from build123d import *

# Parameters (mm, degrees)
SKETCH5_W            = 10
SKETCH5_H            = 100
BOSS_EXTRUDE5_DEPTH  = 3
M3_CLEARANCE_HOLE1_D = 3.6
SKETCH8_R            = 1.75
CUT_EXTRUDE1_DEPTH   = 249.962542564
SKETCH10_W           = 10
SKETCH10_H           = 50
SKETCH10_R           = 1.75
BOSS_EXTRUDE6_DEPTH  = 3
SKETCH11_R           = 1.75
CUT_EXTRUDE2_DEPTH   = 249.962542564


with BuildPart() as part:
    # Sketch5 → Boss-Extrude5 (new body)
    with BuildSketch(Plane(origin=(0, 0, 0), x_dir=(1, 0, 0), z_dir=(0, 1, 0))):
        with Locations((-5, 86)):
            Rectangle(SKETCH5_W, SKETCH5_H)
        Polygon((0, 0), (35, 0), (35, 235.74), (0, 235.74), (0, 136), (0, 36), align=None)
        Polygon((70, 0), (70, 36), (70, 136), (70, 235.74), (35, 235.74), (35, 0), align=None)
        with Locations((75, 86)):
            Rectangle(SKETCH5_W, SKETCH5_H)
    extrude(amount=BOSS_EXTRUDE5_DEPTH)

    # M3 Clearance Hole1 (through all)
    with Locations(Plane(origin=(0, 3, 0), x_dir=(1, 0, 0), z_dir=(0, 1, 0))):
        with Locations((76.5, 50.420635549), (76.5, 42.420635549)):
            m3_clearance_hole1 = Hole(M3_CLEARANCE_HOLE1_D / 2)

    # Sketch8 → Cut-Extrude1 (cut, through all)
    with BuildSketch(Plane(origin=(0, 3, 0), x_dir=(1, 0, 0), z_dir=(0, 1, 0))):
        with Locations(Location((76.5, 58.420635549, 0), (0, 0, 270))):
            Circle(SKETCH8_R)
        with Locations(Location((76.5, 66.420635549, 0), (0, 0, 270))):
            Circle(SKETCH8_R)
        with Locations(Location((76.5, 74.420635549, 0), (0, 0, 270))):
            Circle(SKETCH8_R)
        with Locations(Location((76.5, 82.420635549, 0), (0, 0, 270))):
            Circle(SKETCH8_R)
        with Locations(Location((68.5, 58.420635549, 0), (0, 0, 270))):
            Circle(SKETCH8_R)
        with Locations(Location((68.5, 66.420635549, 0), (0, 0, 270))):
            Circle(SKETCH8_R)
        with Locations(Location((68.5, 74.420635549, 0), (0, 0, 270))):
            Circle(SKETCH8_R)
        with Locations(Location((68.5, 82.420635549, 0), (0, 0, 270))):
            Circle(SKETCH8_R)
        with Locations(Location((68.5, 90.420635549, 0), (0, 0, 270))):
            Circle(SKETCH8_R)
        with Locations(Location((76.5, 90.420635549, 0), (0, 0, 270))):
            Circle(SKETCH8_R)
        with Locations(Location((76.5, 98.420635549, 0), (0, 0, 270))):
            Circle(SKETCH8_R)
        with Locations(Location((68.5, 98.420635549, 0), (0, 0, 270))):
            Circle(SKETCH8_R)
        with Locations(Location((68.5, 106.420635549, 0), (0, 0, 270))):
            Circle(SKETCH8_R)
        with Locations(Location((76.5, 106.420635549, 0), (0, 0, 270))):
            Circle(SKETCH8_R)
        with Locations(Location((68.5, 114.420635549, 0), (0, 0, 270))):
            Circle(SKETCH8_R)
        with Locations(Location((76.5, 114.420635549, 0), (0, 0, 270))):
            Circle(SKETCH8_R)
        with Locations(Location((68.5, 122.420635549, 0), (0, 0, 270))):
            Circle(SKETCH8_R)
        with Locations(Location((76.5, 122.420635549, 0), (0, 0, 270))):
            Circle(SKETCH8_R)
        with Locations(Location((76.5, 130.420635549, 0), (0, 0, 270))):
            Circle(SKETCH8_R)
        with Locations(Location((68.5, 130.420635549, 0), (0, 0, 270))):
            Circle(SKETCH8_R)
    cut_extrude1 = extrude(amount=-CUT_EXTRUDE1_DEPTH, mode=Mode.SUBTRACT)

    # Sketch10 → Boss-Extrude6 (add)
    with BuildSketch(Plane.XZ):
        with Locations((75, -207.420635549)):
            Rectangle(SKETCH10_W, SKETCH10_H)
        with Locations(Location((76.5, -186.420635549, 0), (0, 0, 270))):
            Circle(SKETCH10_R, mode=Mode.SUBTRACT)
        with Locations(Location((76.5, -194.420635549, 0), (0, 0, 270))):
            Circle(SKETCH10_R, mode=Mode.SUBTRACT)
        with Locations(Location((76.5, -202.420635549, 0), (0, 0, 270))):
            Circle(SKETCH10_R, mode=Mode.SUBTRACT)
        with Locations(Location((76.5, -210.420635549, 0), (0, 0, 270))):
            Circle(SKETCH10_R, mode=Mode.SUBTRACT)
        with Locations(Location((76.5, -218.420635549, 0), (0, 0, 270))):
            Circle(SKETCH10_R, mode=Mode.SUBTRACT)
        with Locations(Location((76.5, -226.420635549, 0), (0, 0, 270))):
            Circle(SKETCH10_R, mode=Mode.SUBTRACT)
    boss_extrude6 = extrude(amount=-BOSS_EXTRUDE6_DEPTH)

    # Sketch11 → Cut-Extrude2 (cut, through all)
    with BuildSketch(Plane(origin=(0, 3, 0), x_dir=(1, 0, 0), z_dir=(0, 1, 0))):
        with Locations(Location((68.5, 226.886570254, 0), (0, 0, 270))):
            Circle(SKETCH11_R)
        with Locations(Location((68.5, 218.886570254, 0), (0, 0, 270))):
            Circle(SKETCH11_R)
        with Locations(Location((68.5, 210.886570254, 0), (0, 0, 270))):
            Circle(SKETCH11_R)
        with Locations(Location((68.5, 202.886570254, 0), (0, 0, 270))):
            Circle(SKETCH11_R)
        with Locations(Location((68.5, 194.886570254, 0), (0, 0, 270))):
            Circle(SKETCH11_R)
        with Locations(Location((68.5, 186.886570254, 0), (0, 0, 270))):
            Circle(SKETCH11_R)
    cut_extrude2 = extrude(amount=-CUT_EXTRUDE2_DEPTH, mode=Mode.SUBTRACT)

    # Mirror1: M3 Clearance Hole1, Cut-Extrude1, Boss-Extrude6, Cut-Extrude2 across plane
    add(m3_clearance_hole1.mirror(Plane.ZY.offset(-35)), mode=Mode.SUBTRACT)
    add(cut_extrude1.mirror(Plane.ZY.offset(-35)), mode=Mode.SUBTRACT)
    add(boss_extrude6.mirror(Plane.ZY.offset(-35)))
    add(cut_extrude2.mirror(Plane.ZY.offset(-35)), mode=Mode.SUBTRACT)


solid = part.part
Part model, mm, in its own coordinate system. Coordinates: 2 decimals unless noted, no trailing zeros. Loops run counter-clockwise (first coordinate to the right, second up) from the corner with the lowest first, then second, coordinate; pieces in that order, holes last. Notation, with made-up numbers: M 37,-26 L 67,-26 A19 ccw 67,-2 Z; hole C -2,-11.5 d8. An arc over 180 degrees is marked long. Use a Markdown table: item, result. Add a question column.
Q1. Probe L1, parallel to X at y = 1.05, z = -186.5; L2, parallel to Z at x = -2, y = 1.3; L3, parallel to X at y = 1.6, z = -169. List the from-to ranges inside material, lowest first.
Q2. Cut at A-A (z = -30). Write the cut outline in (x, y), and give its area (3 significant figures).
Q3. Pin check, flat tip, straight feed: P1, Ø0.9, axis at x = 73.5, y = 2, coming from the -Z side. Stop position of the tip, or through.
Q4. Cut at B-B (y = 0.5). Give the number of separate pieces and of enclosed holes in the cut face, and give its area (3 significant figures).
Worked out:
| question | item | result |
|---|---|---|
| 1 | L1 | x = -10 to -8.25, -4.75 to -0.21, 3.21 to 66.79, 70.21 to 74.75, 78.25 to 80 |
| 1 | L2 | z = -232.42 to -182.42, -136 to -36 |
| 1 | L3 | x = 0 to 70 |
| 2 | outline | M 0,0 L 70,0 L 70,3 L 0,3 Z |
| 2 | area | 210 mm2 |
| 3 | P1 | stops at z = -232.42 |
| 4 | separate pieces | 1 |
| 4 | enclosed holes | 68 |
| 4 | area | 18,800 mm2 |
